The model under review builds one solid part; all positions refer to its coordinate system, in mm. A direction names the side the tool comes from. Coordinates: 2 decimals unless noted, no trailing zeros. Loops run counter-clockwise (first coordinate to the right, second up) from the corner with the lowest first, then second, coordinate; pieces in that order, holes last. Notation, with made-up numbers: (-6.5, 29.25) - (17.5, 29.25) arc R21 cw to (17.5, 63.25) - close; hole circle Ø10 at (2.25, -28). An arc over 180 degrees is marked (long way). Use a Markdown table: item, result. Add a question column.
1) For faces 4 (the flat face through (-30.481, 31, -17)), 5 (the flat face through (-1, -1, -17)), 6 (the flat face through (31, -30.481, -17)), 7 (the flat face through (-6.395, -6.919, -16.762)), list the 3-axis set-ups (+Z, -Z, +X, -X, +Y, -Y) from which the entire face can be reached by the end or side of a thin tool; tool diameter is ignored.
2) To check wall thickness, follow L1, parallel to X at y = -36.25, z = -17; L2, parallel to Y at x = 7.5, z = -13.5. State the ranges of each line that lie inside material, in increasing order. Write a range as [from, to].
3) Add section C-C, the plane x = 7. Give the boundary of the cut face in (y, z).
4) Clearance check with flat-ended pins moving along their axes: pin 1 (11.5 mm diameter, centred on y = -18.481, z = -17, fed in from -X); pin 2 (14.5 mm diameter, centred on x = 21.519, z = -17, fed in from +Y); pin 3 (1 mm diameter, centred on y = 26.5, z = -8.5, fed in from +X); pin 4 (12 mm diameter, centred on y = -20, z = -27.5, fed in from +X). State where each tip first meets the part, or that it passes through.
5) Add section A-A, the plane z = -5.5. Give the boundary of the cut face in (x, y), and give its area (3 significant figures).
6) Add section B-B, the plane y = -22. Give the boundary of the cut face in (x, z).
7) The part is to be moulded in two halves that separate along Z. For faces 1 (the cylindrical face through (-34.43, -21.52, -20.32)), 2 (the flat face through (-30.481, -9, -17)), 3 (the flat face through (-3, -8, -34)), say which applies: pulls with the +Z half, pulls with the -Z half, needs draft (parallel to the pull), parting line crosses it, or undercut.
8) Add section D-D, the plane y = -33. Give the boundary of the cut face in (x, z), and give its area (3 significant figures).
Autodesk Inventor part; units mm, degrees
ref_plane "Work Plane1" through (-30.481, -38.481, 0) normal (-1, 0, 0) x (0, 0, 1)
ref_plane "Work Plane2" through (-38.481, -30.481, 0) normal (0, -1, 0) x (1, 0, 0)
ref_plane "YZ Plane" through (0, 0, 0) normal (1, 0, 0) x (0, 1, 0)
sketch "Sketch1" plane through (0, 0, 0) normal (0, 0, 1) x (1, 0, 0)
  line L0 (-38.481, 38.481) -> (38.481, 38.481)
  line L1 (38.481, 38.481) -> (38.481, -38.481)
  line L2 (38.481, -38.481) -> (-38.481, -38.481)
  line L3 (-38.481, -38.481) -> (-38.481, 38.481)
  point P0 (0, 0)
  dimension "d0" = 76.962
  dimension "d1" = 76.962
  dimension "d2" = 38.481
  dimension "d3" = 38.481
extrude "Extrusion1" add sketch "Sketch1" against normal blind 34
sketch "Sketch2" plane through (0, 0, 0) normal (0, 0, 1) x (1, 0, 0)
  line L0 (-38.481, 38.481) -> (38.481, 38.481)
  line L1 (-38.481, -38.481) -> (-38.481, 38.481)
  line L2 (38.481, -38.481) -> (-38.481, -38.481)
  line L3 (38.481, 38.481) -> (38.481, -38.481)
  line L4 (-30.481, 38.481) -> (-30.481, 28.481)
  line L5 (-30.481, 28.481) -> (28.481, -30.481)
  line L6 (28.481, -30.481) -> (38.481, -30.481)
  line L7 (-30.481, 17.1673) -> (-30.481, -30.481)
  line L8 (-30.481, -30.481) -> (17.1673, -30.481)
  line L9 (17.1673, -30.481) -> (-30.481, 17.1673)
  dimension "d6" = 8
  dimension "d7" = 8
  dimension "d8" = 10
  dimension "d10" = 135
  dimension "d11" = 8
extrude "Extrusion2" cut sketch "Sketch2" against normal through all contours L0 L3 L6 L5 L4 | L9 L8 L7
fillet "Fillet1" radius 2 1 edges at (-30.481, -30.481, -17)
fillet "Fillet1" radius 1 4 edges at (-30.481, 38.481, -17) (-30.481, 28.481, -17) (28.481, -30.481, -17) (38.481, -30.481, -17)
fillet "Fillet1" radius 3 2 edges at (-30.481, 17.1673, -17) (17.1673, -30.481, -17)
sketch "Sketch3" plane through (-38.481, -38.481, 0) normal (-1, 0, 0) x (0, 0, 1)
  line L0 (0, 0) -> (-34, 0)
  line L1 (0, 0) -> (0, 76.962)
  point P0 (-17, 60)
  point P1 (-17, 20)
  dimension "d17" = 17
  dimension "d18" = 20
  dimension "d19" = 40
hole "Hole1" at (-38.481, 21.519, -17) at (-38.481, -18.481, -17) direction (1, 0, 0) diameter 9 end through all
sketch "Sketch4" plane through (-38.481, -38.481, 0) normal (0, -1, 0) x (1, 0, 0)
  line L0 (0, -34) -> (76.962, -34)
  line L1 (0, 0) -> (0, -34)
  point P0 (20, -17)
  point P1 (60, -17)
  dimension "d27" = 17
  dimension "d28" = 20
  dimension "d29" = 40
hole "Hole2" at (-18.481, -38.481, -17) at (21.519, -38.481, -17) direction (0, 1, 0) diameter 9 end through all
ref_plane "Work Plane1" through (-30.481, -38.481, 0) normal (-1, 0, 0) x (0, 0, 1)
ref_plane "Work Plane2" through (-38.481, -30.481, 0) normal (0, -1, 0) x (1, 0, 0)
sketch "Sketch5" plane through (-30.481, -38.481, 0) normal (-1, 0, 0) x (0, 0, 1)
  arc A0 (-13.2711, 57.481) -> (-20.7289, 57.481) centre (-17, 60) ccw
  circle A1 centre (-17, 60) radius 4.5
  circle A2 centre (-17, 60) radius 7.5
  dimension "d39" = 15
extrude "Extrusion3" cut sketch "Sketch5" against normal through all
sketch "Sketch6" plane through (-38.481, -30.481, 0) normal (0, -1, 0) x (1, 0, 0)
  arc A0 (57.481, -20.7289) -> (57.481, -13.2711) centre (60, -17) ccw
  circle A1 centre (60, -17) radius 4.5
  circle A2 centre (60, -17) radius 7.5
  dimension "d42" = 15
extrude "Extrusion4" cut sketch "Sketch6" against normal through all
ref_plane "OffsetPlane" through (0, 0, -17) normal (0, 0, 1) x (1, 0, 0)
properties part number "20-102" material "Alluminio - 6061"
From the geometry:
| question | item | result |
|---|---|---|
| 1 | face 4 | +X |
| 1 | face 5 | +Z, -Z, +X, +Y |
| 1 | face 6 | +Y |
| 1 | face 7 | +Z, -Z |
| 2 | L1 | x = [-38.48, -22.98], [-13.98, 17.02], [26.02, 38.48] |
| 2 | L2 | y = [-38.48, -30.48], [-15.65, -9.5] |
| 3 | outline | (-38.48, -34) - (-30.48, -34) - (-30.48, 0) - (-38.48, 0) - close; (-20.31, -34) - (-9, -34) - (-9, 0) - (-20.31, 0) - (-20.31, -12.89) arc R4.5 cw (long way) to (-20.31, -21.11) - close |
| 4 | pin 1 | stops at x = -38.48 |
| 4 | pin 2 | stops at y = -30.48 |
| 4 | pin 3 | stops at x = -28 |
| 4 | pin 4 | stops at x = 24 |
| 5 | outline | (-38.48, -38.48) - (38.48, -38.48) - (38.48, -31.48) arc R1 ccw to (37.48, -30.48) - (28.9, -30.48) arc R1 cw to (28.19, -30.19) - (-30.19, 28.19) arc R1 cw to (-30.48, 28.9) - (-30.48, 37.48) arc R1 ccw to (-31.48, 38.48) - (-38.48, 38.48) - close; hole (-30.48, -28.48) arc R2 ccw to (-28.48, -30.48) - (9.92, -30.48) arc R3 ccw to (12.05, -25.36) - (-25.36, 12.05) arc R3 ccw to (-30.48, 9.92) - close |
| 5 | area | 1,790 mm^2 |
| 6 | outline | (-38.48, -34) - (-30.48, -34) - (-30.48, -19.8) - (-38.48, -19.8) - close; (-38.48, -14.2) - (-30.48, -14.2) - (-30.48, 0) - (-38.48, 0) - close; (8.69, -34) - (20, -34) - (20, -24.34) arc R7.5 cw to (14.56, -19.8) - (8.69, -19.8) - close; (8.69, -14.2) - (14.56, -14.2) arc R7.5 cw to (20, -9.66) - (20, 0) - (8.69, 0) - close |
| 7 | face 1 | undercut |
| 7 | face 2 | needs draft |
| 7 | face 3 | pulls with the -Z half |
| 8 | outline | (-38.48, -34) - (38.48, -34) - (38.48, 0) - (-38.48, 0) - close; hole circle Ø9 at (-18.48, -17); hole circle Ø9 at (21.52, -17) |
| 8 | area | 2,490 mm^2 |
